```python
from build123d import *

# Parameters (mm, degrees)
SKETCH_1_W          = 15
SKETCH_1_H          = 21
SKETCH_1_W_2        = 12
SKETCH_1_H_2        = 18
EXTRUDE_1_DEPTH     = 260
SKETCH_4_R          = 1.5
CUT_EXTRUDE_2_DEPTH = 261.643914182
SKETCH_5_R          = 1.5
CUT_EXTRUDE_3_DEPTH = 261.954497949


with BuildPart() as part:
    # 草图1 → 拉伸-薄壁1 (new body)
    with BuildSketch(Plane(origin=(0, 0, 0), x_dir=(1, 0, 0), z_dir=(0, 1, 0))):
        Rectangle(SKETCH_1_W, SKETCH_1_H)
        Rectangle(SKETCH_1_W_2, SKETCH_1_H_2, mode=Mode.SUBTRACT)
    extrude(amount=EXTRUDE_1_DEPTH)

    # 草图4 → 切除-拉伸2 (cut, through all)
    with BuildSketch(Plane(origin=(7.5, 0, 0), x_dir=(0, 0, -1), z_dir=(1, 0, 0))):
        with Locations((0, 252.5)):
            Circle(SKETCH_4_R)
        with Locations((0, 232.5)):
            Circle(SKETCH_4_R)
        with Locations((0, 27.5)):
            Circle(SKETCH_4_R)
        with Locations((0, 7.5)):
            Circle(SKETCH_4_R)
    extrude(amount=-CUT_EXTRUDE_2_DEPTH, mode=Mode.SUBTRACT)

    # 草图5 → 切除-拉伸3 (cut, through all)
    with BuildSketch(Plane.XY.offset(10.5)):
        with Locations((0, 40)):
            Circle(SKETCH_5_R)
        with Locations((0, 60)):
            Circle(SKETCH_5_R)
        with Locations((0, 120)):
            Circle(SKETCH_5_R)
        with Locations((0, 140)):
            Circle(SKETCH_5_R)
    extrude(amount=-CUT_EXTRUDE_3_DEPTH, mode=Mode.SUBTRACT)


solid = part.part
```
Input: part model. Units: mm. Frame: model coordinates. A direction names the side the tool comes from. Give positions to 0.01 mm unless a question says otherwise; leave off trailing zeros. Write each loop counter-clockwise with the first axis right and the second up, starting at its lowest first coordinate (ties: lowest second). Pieces come first, ordered by that corner, then holes. Notation, with made-up numbers: (15, 89.5) - (58, 89.5) arc R20 cw to (58, 125.5) - close; hole circle Ø8 at (56.25, 17). An arc over 180 degrees is marked (long way). Write item = value, one per line. Start each with the question number.
1. Mould query, pull axis X, two halves, no side actions, for faces 1 (the flat face through (-6, 128, 0)), 2 (the flat face through (7.5, 128, 0)), 3 (the flat face through (0, 128, 10.5)), 4 (the flat face through (0, 128, 9)). Classes: released by +X, released by -X, zero draft, split by the parting line, or undercut.
2. Section query A-A, the plane y = 104.5. Output: boundary loops of the cut face in (x, z).
3. Ray query, L1, parallel to Y at x = 7.2, z = 0; L2, parallel to Y at x = 0, z = -10; L3, parallel to Z at x = -5.75, y = 217. Return the intervals inside material, ascending.
4. Access query for faces 5 (the flat face through (6, 128, 0)), 6 (the flat face through (-7, 0, 0)). Directions: +Z, -Z, +X, -X, +Y, -Y. A direction counts if a zero-diameter tool reaches every point of the face in a straight line with its end or side. Return the directions, or none.
5. First-contact query: pin 1 Ø2.5 at (x, y) = (0, 60) entering from +Z; pin 2 Ø6 at (x, z) = (-3, -7) entering from -Y. Flat tips, straight axial feed; report the tip coordinate or a pass-through.
Check sheet entries:
q1.face_1 = undercut
q1.face_2 = released by +X
q1.face_3 = zero draft
q1.face_4 = undercut
q2.outline = (-7.5, -10.5) - (7.5, -10.5) - (7.5, 10.5) - (-7.5, 10.5) - close; hole (-6, -9) - (6, -9) - (6, 9) - (-6, 9) - close
q3.L1 = 0 to 6, 9 to 26, 29 to 231, 234 to 251, 254 to 260
q3.L2 = 0 to 38.5, 41.5 to 58.5, 61.5 to 118.5, 121.5 to 138.5, 141.5 to 260
q3.L3 = -10.5 to -9, 9 to 10.5
q4.face_5 = +Y, -Y
q4.face_6 = +Z, -Z, +X, -X, -Y
q5.pin_1 = through
q5.pin_2 = 0
